from build123d import *

# Parameters (mm, degrees)
SKETCH2_R           = 1.905
BOSS_EXTRUDE1_DEPTH = 11.1125


with BuildPart() as part:
    # Sketch2 → Boss-Extrude1 (new body)
    with BuildSketch(Plane(origin=(0, 0, 0), x_dir=(1, 0, 0), z_dir=(0, 1, 0))):
        with BuildLine():
            Line((-16.652885777, 7.290524058), (-15.327609815, 12.747542729))
            ThreePointArc((-15.327609815, 12.747542729), (-13.558199469, 18.045958382), (-18.96031801, 16.624291517))
            Line((-18.96031801, 16.624291517), (-21.65906801, 5.511791517))
            ThreePointArc((-21.65906801, 5.511791517), (-21.726249777, 5.139819704), (-21.74875, 4.7625))
            Line((-21.74875, 4.7625), (-21.74875, -4.397375))
            ThreePointArc((-21.74875, -4.397375), (-21.726434075, -4.773151689), (-21.659800003, -5.143645982))
            Line((-21.659800003, -5.143645982), (-18.961050003, -16.303770982))
            ThreePointArc((-18.961050003, -16.303770982), (-13.540192666, -17.709080747), (-15.382866617, -12.420872873))
            Line((-15.382866617, -12.420872873), (-16.702800144, -6.962559523))
            ThreePointArc((-16.702800144, -6.962559523), (-15.743476975, -5.836186872), (-15.39875, -4.397375))
            Line((-15.39875, -4.397375), (-15.39875, -3.175))
            Line((-15.39875, -3.175), (15.39875, -3.175))
            Line((15.39875, -3.175), (15.39875, -4.397375))
            ThreePointArc((15.39875, -4.397375), (15.743476975, -5.836186872), (16.702800144, -6.962559523))
            Line((16.702800144, -6.962559523), (15.382866617, -12.420872873))
            ThreePointArc((15.382866617, -12.420872873), (13.540192666, -17.709080747), (18.961050003, -16.303770982))
            Line((18.961050003, -16.303770982), (21.659800003, -5.143645982))
            ThreePointArc((21.659800003, -5.143645982), (21.726434075, -4.773151689), (21.74875, -4.397375))
            Line((21.74875, -4.397375), (21.74875, 4.7625))
            ThreePointArc((21.74875, 4.7625), (21.726249777, 5.139819704), (21.65906801, 5.511791517))
            Line((21.65906801, 5.511791517), (18.96031801, 16.624291517))
            ThreePointArc((18.96031801, 16.624291517), (13.558199469, 18.045958382), (15.327609815, 12.747542729))
            Line((15.327609815, 12.747542729), (16.652885777, 7.290524058))
            ThreePointArc((16.652885777, 7.290524058), (15.72951294, 6.173506926), (15.39875, 4.7625))
            Line((15.39875, 4.7625), (15.39875, 3.175))
            Line((15.39875, 3.175), (-15.39875, 3.175))
            Line((-15.39875, 3.175), (-15.39875, 4.7625))
            ThreePointArc((-15.39875, 4.7625), (-15.72951294, 6.173506926), (-16.652885777, 7.290524058))
        make_face()
        with Locations(Location((-15.875, 15.875, 0), (0, 0, 270))):
            Circle(SKETCH2_R, mode=Mode.SUBTRACT)
        with Locations(Location((-18.57375, 4.7625, 0), (0, 0, 270))):
            Circle(SKETCH2_R, mode=Mode.SUBTRACT)
        with Locations(Location((-18.57375, -4.397375, 0), (0, 0, 90))):
            Circle(SKETCH2_R, mode=Mode.SUBTRACT)
        with Locations(Location((-15.875, -15.5575, 0), (0, 0, 90))):
            Circle(SKETCH2_R, mode=Mode.SUBTRACT)
        with Locations(Location((15.875, -15.5575, 0), (0, 0, 270))):
            Circle(SKETCH2_R, mode=Mode.SUBTRACT)
        with Locations(Location((18.57375, -4.397375, 0), (0, 0, 270))):
            Circle(SKETCH2_R, mode=Mode.SUBTRACT)
        with Locations(Location((18.57375, 4.7625, 0), (0, 0, 90))):
            Circle(SKETCH2_R, mode=Mode.SUBTRACT)
        with Locations(Location((15.875, 15.875, 0), (0, 0, 90))):
            Circle(SKETCH2_R, mode=Mode.SUBTRACT)
    extrude(amount=BOSS_EXTRUDE1_DEPTH)


solid = part.part
Here's how the part is built. I have some questions about the finished solid (model axes, mm). A direction names the side the tool comes from. Round coordinates to 2 decimals unless told otherwise and drop trailing zeros. Write each loop counter-clockwise with the first axis right and the second up, starting at its lowest first coordinate (ties: lowest second). Pieces come first, ordered by that corner, then holes.
1. For faces 4 (the cylindrical face through (15.739, 5.478, -6.192)), 5 (the flat face through (0, 0, 0)), which set-ups out of +Z, -Z, +X, -X, +Y, -Y let a thin tool reach every point of the face, with its end or its side?
2. Will these pins go through, and if not, where does the flat tip stop? pin 1 Ø5.5 at (x, y) = (7, 8) entering from -Z (3 decimals); pin 2 Ø2 at (x, y) = (-3, 7.5) entering from +Z (3 decimals).
3. I need wall thicknesses on L1, parallel to X at y = 0.5, z = 6; L2, parallel to X at y = 7.5, z = -14.5; L3, parallel to Z at x = -1.5, y = 7.5 (3 decimals). Which ranges of each line are inside material? Lowest first, please.
4. Suppose I cut it at D-D (y = 6.25). State how many separate pieces and enclosed holes the cut face has, and give its area (3 significant figures).
5. If we mould it in two halves opening along Z, with no side actions, what happens to faces 1 (the flat face through (16.052, 5.478, 9.654)), 2 (the flat face through (20.33, 5.48, -10.99)), 3 (the flat face through (0, 11.112, 0))? For each: released by +Z, released by -Z, zero draft, split by the parting line, or undercut.
6. Suppose I cut it at A-A (z = 11). List the corners of the cut face in (x, y) for me.
7. Suppose I cut it at B-B (z = -4). List the corners of the cut face in (x, y) for me.
8. Suppose I cut it at C-C (x = 6.5). List the corners of the cut face in (y, z) for me (1 decimal).
Answer sheet:
1. face 4: +Y, -Y
1. face 5: +Z, -Z, +X, -X, -Y
2. pin 1: stops at z = -3.175
2. pin 2: stops at z = 3.175
3. L1: x = -21.45 to -19.6, -17.54 to -15.83, 15.83 to 17.54, 19.6 to 21.45
3. L2: x = -19.48 to -17.19, -14.56 to -13.01, 13.01 to 14.56, 17.19 to 19.48
3. L3: z = -3.175 to 3.175
4. separate pieces: 1
4. enclosed holes: 8
4. area: 519 mm2
5. face 1: undercut
5. face 2: released by -Z
5. face 3: zero draft
6. outline: (-20.24, 0) - (-15.73, 0) - (-15.73, 11.11) - (-20.24, 11.11) - close; (15.73, 0) - (20.24, 0) - (20.24, 11.11) - (15.73, 11.11) - close
7. outline: (-21.75, 0) - (-20.32, 0) - (-20.32, 11.11) - (-21.75, 11.11) - close; (-16.83, 0) - (-15.4, 0) - (-15.4, 11.11) - (-16.83, 11.11) - close; (15.4, 0) - (16.83, 0) - (16.83, 11.11) - (15.4, 11.11) - close; (20.32, 0) - (21.75, 0) - (21.75, 11.11) - (20.32, 11.11) - close
8. outline: (0, -3.2) - (11.1, -3.2) - (11.1, 3.2) - (0, 3.2) - close
